Design review of the part shown in the three views and the two pictorial views. Dimensions are in mm from the part's minimum x, y and z. Coordinates: 2 decimals unless noted, no trailing zeros. Loops run counter-clockwise (first coordinate to the right, second up) from the corner with the lowest first, then second, coordinate; pieces in that order, holes last. Notation, with made-up numbers: M 56.25,7.25 L 91.25,7.25 A14 cw 91.25,33.25 Z; hole C -12,-29.5 d11. An arc over 180 degrees is marked long. Put each result on its own line as item: value. Start each with the question number.
(1) For probe 1 along Y at (x, z) = (13, 8); probe 2 along X at (y, z) = (11.25, 14.75); probe 3 along X at (y, z) = (5.25, 16.25), list the stretches that pass through material, from the lowest coordinate up. Write a range as [from, to].
(2) The part is to be moulded in two halves that separate along X. For the marked faces 1 and 2, say which applies: +X half, -X half, draft (parallel to the pull), parting line (faces both ways), or undercut.
(3) Clearance check with flat-ended pins moving along their axes: pin 1 (4 mm diameter, centred on y = 17, z = 13, fed in from +X); pin 2 (5 mm diameter, centred on x = 22, z = 9.5, fed in from -Y); pin 3 (1 mm diameter, centred on x = 19.5, z = 4, fed in from -Y). State where each tip first meets the part, or that it passes through.
(4) Take a section at C-C, the plane z = 6. Give the boundary of the cut face in (x, y), then the cut area to 3 significant figures.
(5) Take a section at A-A, the plane y = 13. Give the boundary of the cut face in (x, z), then the cut area to 3 significant figures.
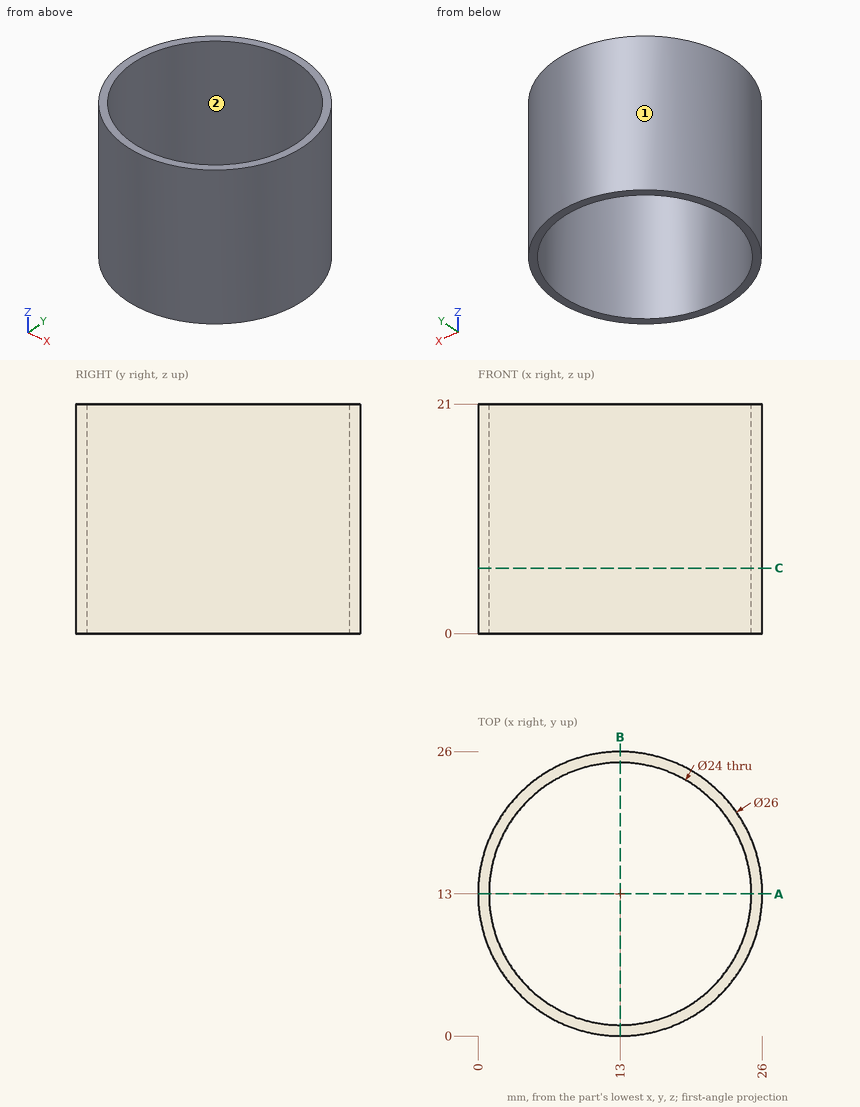
Computed values:
1. probe 1: y = [0, 1], [25, 26]
1. probe 2: x = [0.12, 1.13], [24.87, 25.88]
1. probe 3: x = [2.56, 3.84], [22.16, 23.44]
2. face 1: parting line
2. face 2: undercut
3. pin 1: stops at x = 25.85
3. pin 2: stops at y = 1.74
3. pin 3: stops at y = 1.47
4. outline: C 13,13 d26; hole C 13,13 d24
4. area: 78.5 mm^2
5. outline: M 0,0 L 1,0 L 1,21 L 0,21 Z; M 25,0 L 26,0 L 26,21 L 25,21 Z
5. area: 42.0 mm^2
